from build123d import *

# Parameters (mm, degrees)
SKETCH1_W           = 56
SKETCH1_H           = 41
BOSS_EXTRUDE1_DEPTH = 2.5
SKETCH2_W           = 51.5
SKETCH2_H           = 39.5
CUT_EXTRUDE1_DEPTH  = 1.5
SKETCH3_W           = 3.7
SKETCH3_H           = 35
CUT_EXTRUDE2_DEPTH  = 1.5


with BuildPart() as part:
    # Sketch1 → Boss-Extrude1 (new body)
    with BuildSketch(Plane.XY):
        with Locations((0.145813854, -9.904151416)):
            Rectangle(SKETCH1_W, SKETCH1_H)
    extrude(amount=BOSS_EXTRUDE1_DEPTH)

    # Sketch2 → Cut-Extrude1 (cut)
    with BuildSketch(Plane.XY.offset(2.5)):
        with Locations((1.595813854, -9.904151416)):
            Rectangle(SKETCH2_W, SKETCH2_H)
    extrude(amount=-CUT_EXTRUDE1_DEPTH, mode=Mode.SUBTRACT)

    # Sketch3 → Cut-Extrude2 (cut)
    with BuildSketch(Plane.XY.offset(2.5)):
        with Locations((-26.004186146, -9.904151416)):
            Rectangle(SKETCH3_W, SKETCH3_H)
    extrude(amount=-CUT_EXTRUDE2_DEPTH, mode=Mode.SUBTRACT)


solid = part.part
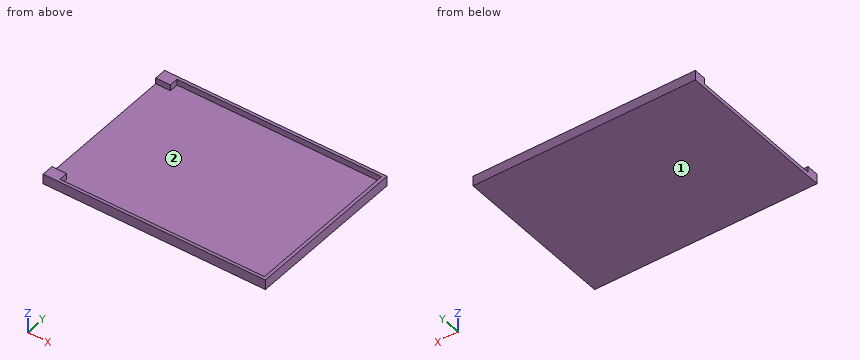
Source: CAD feature listing. Evaluate the final solid. Frame: model axes, mm. Face numbers are marked on the shaded views. Give positions to 0.01 mm unless a question says otherwise; leave off trailing zeros. Loops run counter-clockwise (first coordinate to the right, second up) from the corner with the lowest first, then second, coordinate; pieces in that order, holes last. Notation, with made-up numbers: (-14, 33) -> (-2, 33) arc R23 ccw to (-2, 58) -> close; hole circle Ø7 at (-28.5, 20.25). An arc over 180 degrees is marked (long way). Use a Markdown table: item, result. Add a question column.
1) Line query: line 1 along Y through (x, z) = (17, 1.95); line 2 along X through (y, z) = (-6.5, 1.5); line 3 along Z through (x, y) = (-25, 0). Output: solid intervals per line, ascending. Write a range as [from, to].
2) Section query B-B, the plane x = 18. Return the cut outline in (y, z), then the cut area to 4 significant figures.
3) Section query C-C, the plane y = -24.5. Return the cut outline in (x, z).
4) Section query A-A, the plane z = 1.5. Return the cut outline in (x, y), then the cut area to 3 significant figures.
5) Pull-direction query (Y, two-part tool) for the marked faces 1 and 2; classes: +Y half, -Y half, draft (parallel to the pull), parting line (faces both ways), or undercut.
6) First-contact query: pin 1 (8 mm diameter, centred on x = 10, y = -5.5, fed in from +Z). Flat tip, straight axial feed; report the tip coordinate or a pass-through.
Numbers:
| question | item | result |
|---|---|---|
| 1 | line 1 | y = [-30.4, -29.65], [9.85, 10.6] |
| 1 | line 2 | x = [27.35, 28.15] |
| 1 | line 3 | z = [0, 1] |
| 2 | outline | (-30.4, 0) -> (10.6, 0) -> (10.6, 2.5) -> (9.85, 2.5) -> (9.85, 1) -> (-29.65, 1) -> (-29.65, 2.5) -> (-30.4, 2.5) -> close |
| 2 | area | 43.25 mm2 |
| 3 | outline | (-27.85, 0) -> (28.15, 0) -> (28.15, 2.5) -> (27.35, 2.5) -> (27.35, 1) -> (-27.85, 1) -> close |
| 4 | outline | (-27.85, -30.4) -> (28.15, -30.4) -> (28.15, 10.6) -> (-27.85, 10.6) -> (-27.85, 7.6) -> (-24.15, 7.6) -> (-24.15, 9.85) -> (27.35, 9.85) -> (27.35, -29.65) -> (-24.15, -29.65) -> (-24.15, -27.4) -> (-27.85, -27.4) -> close |
| 4 | area | 132 mm2 |
| 5 | face 1 | draft |
| 5 | face 2 | undercut |
| 6 | pin 1 | stops at z = 1 |
